Print and shaded views of the part. All mm, measured from the part's lowest x, y and z. Coordinates: 2 decimals unless noted, no trailing zeros. Order: outer loops, then holes, each group sorted by start corner. A loop starts at its lowest first (then second) coordinate and runs counter-clockwise, first axis right, second up. Notation, with made-up numbers: (70, -14.75) -> (89, -14.75) arc R8 cw to (89, 0.25) -> close; hole circle Ø7 at (89.5, 86). An arc over 180 degrees is marked (long way). Write item = value, one per line. Start each with the question number.
Q1. Flat gauge pins, fed straight in: pin 1 (1.5 mm diameter, centred on y = 92, z = 267.5, fed in from +X); pin 2 (7 mm diameter, centred on x = 287.33, z = 215.13, fed in from +Y); pin 3 (1.5 mm diameter, centred on y = 37.5, z = 279, fed in from +X); pin 4 (1 mm diameter, centred on x = 175, y = 12.5, fed in from -Z). Where does each tip first touch, or does it go through?
Q2. Mould opens along Z. For the marked faces 1, 2 and 3 say: +Z half, -Z half, draft (parallel to the pull), parting line (faces both ways), or undercut.
Q3. Wall check: line 1 (Z direction, x = 98, y = 42) (1 decimal); line 2 (X direction, y = 72, z = 16.25) (1 decimal); line 3 (X direction, y = 59.5, z = 26) (1 decimal). Give the ranges that are in metal, low to high. Write a range as from..to.
Q4. Cut at B-B, the plane x = 157.5. List the corners of the cut face in (y, z), plus the area to 4 significant figures.
Q5. Cut at A-A, the plane z = 157.5. List the corners of the cut face in (x, y), plus the area to 4 significant figures.
Q6. Cut at C-C, the plane y = 101.5. Give the number of separate pieces and of enclosed holes in the cut face, plus the area to 3 significant figures.
Q7. Cut at D-D, the plane x = 16.25. List the corners of the cut face in (y, z) (1 decimal), plus the area to 3 significant figures.
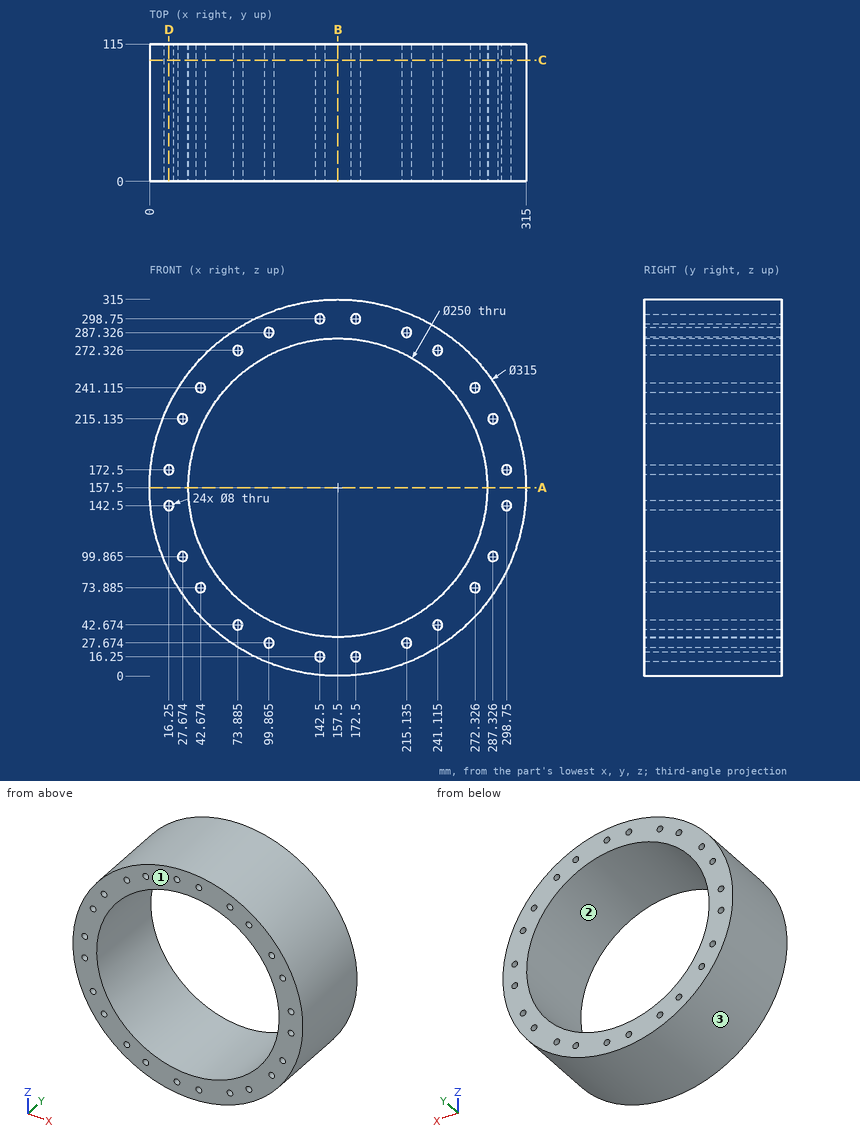
Here are the results:
q1.pin_1 = 270.95
q1.pin_2 = through
q1.pin_3 = 258.62
q1.pin_4 = 0.92
q2.face_1 = draft
q2.face_2 = undercut
q2.face_3 = parting line
q3.line_1 = 11.7..24.1, 31.2..47.6, 267.4..283.8, 290.9..303.3
q3.line_2 = 87.8..138.5, 146.5..168.5, 176.5..227.2
q3.line_3 = 70.8..96.2, 103.5..211.5, 218.8..244.2
q4.outline = (0, 0) -> (115, 0) -> (115, 32.5) -> (0, 32.5) -> close; (0, 282.5) -> (115, 282.5) -> (115, 315) -> (0, 315) -> close
q4.area = 7,475 mm²
q5.outline = (0, 0) -> (32.5, 0) -> (32.5, 115) -> (0, 115) -> close; (282.5, 0) -> (315, 0) -> (315, 115) -> (282.5, 115) -> close
q5.area = 7,475 mm²
q6.separate_pieces = 1
q6.enclosed_holes = 25
q6.area = 27,600 mm²
q7.outline = (0, 87.8) -> (115, 87.8) -> (115, 138.5) -> (0, 138.5) -> close; (0, 146.5) -> (115, 146.5) -> (115, 168.5) -> (0, 168.5) -> close; (0, 176.5) -> (115, 176.5) -> (115, 227.2) -> (0, 227.2) -> close
q7.area = 14,200 mm²
